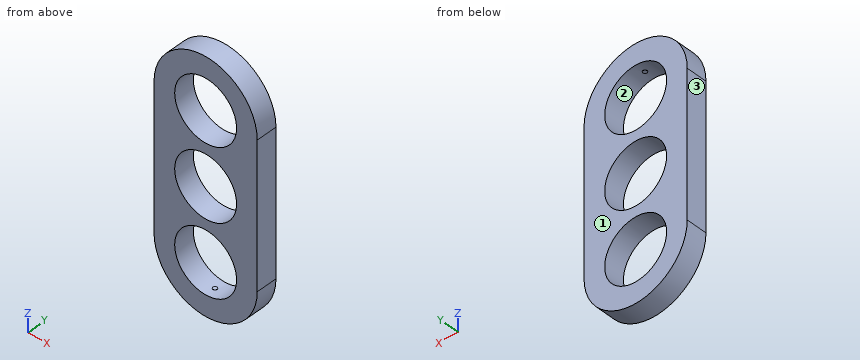
Autodesk Inventor part; units mm, degrees
ref_plane "Plano de trabajo1" through (0, 0, 35) normal (1, 0, 0) x (0, 0, -1)
ref_plane "Plano de trabajo2" through (0, 5, -50) normal (0, 0, 1) x (1, 0, 0)
ref_plane "Plano de trabajo3" through (0, 10, 50) normal (0, 0, 1) x (1, 0, 0)
sketch "Boceto1" plane through (0, 0, 0) normal (0, 1, 0) x (-1, 0, 0)
  line L0 (0, 35) -> (0, -35) construction
  line L1 (25, 35) -> (25, -35)
  line L2 (-25, -35) -> (-25, 35)
  arc A0 (25, 35) -> (-25, 35) centre (0, 35) ccw
  arc A1 (-25, -35) -> (25, -35) centre (0, -35) ccw
  circle A2 centre (0, -35) radius 15
  circle A3 centre (0, 35) radius 15
  line L3 (0, -20) -> (0, -20)
  line L4 (15, -35) -> (-15, -35)
  line L5 (94.5074, 0) -> (-76.0102, 0) construction
  line L6 (15, 35) -> (-15, 35)
  line L7 (15, -35) -> (-15, -35)
  circle A4 centre (0, 0) radius 15
  point P0 (0, 60)
  point P1 (0, -60)
  point P2 (0, -20)
  point P3 (15, 35)
  dimension "largo" = 120
  dimension "ancho" = 50
  dimension "espesor_junta" = 10
  dimension "d3" = 10
  dimension "d6" = 0
  dimension "d12" = 30
extrude "Extrusión3" add sketch "Boceto1" along normal blind 10
ref_plane "Plano de trabajo1" through (0, 0, 35) normal (1, 0, 0) x (0, 0, -1)
sketch "Boceto2" plane through (0, 0, 35) normal (1, 0, 0) x (0, 0, -1)
  line L0 (15, 0) -> (15, 10)
  line L1 (15, 10) -> (20, 10)
  line L2 (20, 10) -> (20, 0)
  line L3 (20, 0) -> (15, 0)
  line L4 (55, 10) -> (55, 0)
  line L5 (55, 0) -> (50, 0)
  line L6 (50, 0) -> (50, 10)
  line L7 (50, 10) -> (55, 10)
  line L8 (95, 10) -> (95, 0)
  line L9 (95, 0) -> (85, 0)
  line L10 (85, 0) -> (85, 10)
  line L11 (85, 10) -> (95, 10)
  line L12 (-25, 0) -> (-25, 10)
  line L13 (-25, 10) -> (-15, 10)
  line L14 (-15, 10) -> (-15, 0)
  line L15 (-15, 0) -> (-25, 0)
  line L16 (-15, 10) -> (-15, 0)
  point P0 (35, 0)
  point P1 (85, 5)
  point P2 (-15, 5)
ref_plane "Plano de trabajo2" through (0, 5, -50) normal (0, 0, 1) x (1, 0, 0)
ref_plane "Plano de trabajo3" through (0, 10, 50) normal (0, 0, 1) x (1, 0, 0)
sketch "Boceto3" plane through (0, 5, -50) normal (0, 0, 1) x (1, 0, 0)
  circle A0 centre (0, 0) radius 1
  point P0 (0, -5)
  dimension "d16" = 2
extrude "Extrusión4" add sketch "Boceto3" along normal blind 0.1
sketch "Boceto4" plane through (0, 10, 50) normal (0, 0, 1) x (1, 0, 0)
  line L0 (-20, -10) -> (-20, 0)
  line L1 (-20, 0) -> (0, 0)
  line L2 (0, 0) -> (0, -10)
  line L3 (20, -10) -> (0, -10)
  line L4 (20, 0) -> (20, -10)
  line L5 (0, 0) -> (20, 0)
  line L6 (0, -10) -> (-20, -10)
  circle A0 centre (0, -5) radius 1
  dimension "d19" = 2
extrude "Extrusión5" add sketch "Boceto4" against normal blind 0.1 contours A0 L2 | L2 A0
equation "\"d3\" = espesor_junta"
equation "\"d15\" = -0.5 * ancho"
properties part number "mod3_3DPrint"
Design review of the part built by this model. Coordinates are the model's own, in mm. Face numbers are marked on the shaded views. Coordinates: 2 decimals unless noted, no trailing zeros. Loops run counter-clockwise (first coordinate to the right, second up) from the corner with the lowest first, then second, coordinate; pieces in that order, holes last. Notation, with made-up numbers: (82, 1.25) -> (91, 1.25) arc R28 ccw to (91, 21.25) -> close; hole circle Ø7 at (88.25, -9). An arc over 180 degrees is marked (long way). Use a Markdown table: item, result. Add a question column.
Item 1: We need section B-B, the plane y = 8.5. Write out the cut boundary in (x, z).
Item 2: Clearance check with flat-ended pins moving along their axes: P1, Ø2, axis at x = -0.5, y = 5.5, coming from the -Z side; P2, Ø1.5, axis at x = -9, y = 4.5, coming from the +Z side; P3, Ø1.5, axis at x = 11.5, z = 29, coming from the +Y side; P4, Ø1.5, axis at x = -16, y = 8, coming from the -Z side. State where each tip first meets the part, or that it passes through.
Item 3: We need section C-C, the plane x = 12.5. Write out the cut boundary in (y, z).
Item 4: We need section D-D, the plane z = -30. Write out the cut boundary in (x, y).
Item 5: Wall thickness on L1, parallel to Z at x = 0, y = 6.75; L2, parallel to X at y = 1, z = 35; L3, parallel to Z at x = 0, y = 5: over which ranges is each line inside the solid? List them lowest first. Write a range as from..to.
Item 6: The part is to be moulded in two halves that separate along X. For the marked faces 1, 2 and 3, say which applies: +X half, -X half, draft (parallel to the pull), parting line (faces both ways), or undercut.
Item 7: We need section A-A, the plane z = 0. Write out the cut boundary in (x, y), and give its area (3 significant figures).
Numbers:
| question | item | result |
|---|---|---|
| 1 | outline | (-25, -35) arc R25 ccw to (25, -35) -> (25, 35) arc R25 ccw to (-25, 35) -> close; hole circle Ø30 at (0, -35); hole circle Ø30 at (0, 0); hole circle Ø30 at (0, 35) |
| 2 | P1 | stops at z = -60 |
| 2 | P2 | stops at z = 58.6 |
| 2 | P3 | passes through |
| 2 | P4 | stops at z = -54.81 |
| 3 | outline | (0, -56.65) -> (10, -56.65) -> (10, -43.29) -> (0, -43.29) -> close; (0, -26.71) -> (10, -26.71) -> (10, -8.29) -> (0, -8.29) -> close; (0, 8.29) -> (10, 8.29) -> (10, 26.71) -> (0, 26.71) -> close; (0, 43.29) -> (10, 43.29) -> (10, 56.65) -> (0, 56.65) -> close |
| 4 | outline | (-25, 0) -> (-14.14, 0) -> (-14.14, 10) -> (-25, 10) -> close; (14.14, 0) -> (25, 0) -> (25, 10) -> (14.14, 10) -> close |
| 5 | L1 | z = -60..-50, -20..-15, 15..20, 50..60 |
| 5 | L2 | x = -25..-15, 15..25 |
| 5 | L3 | z = -60..-49.9, -20..-15, 15..20, 49.9..60 |
| 6 | face 1 | draft |
| 6 | face 2 | undercut |
| 6 | face 3 | -X half |
| 7 | outline | (-25, 0) -> (-15, 0) -> (-15, 10) -> (-25, 10) -> close; (15, 0) -> (25, 0) -> (25, 10) -> (15, 10) -> close |
| 7 | area | 200 mm^2 |
